Autodesk Fusion 360 part; units mm, degrees
cylinder "CylinderPrimitive1" add diameter 18.6 height 24.7 placed x (1, 0, 0) y (0, 0, -1) z (0, 1, 0) at (0, 0, 0)
hole "Hole1" at (0, 24.7, 0) direction (0, -1, 0) diameter 8 depth 10 tip angle 180
hole "Hole2" at (0, 0, 0) direction (0, 1, 0) diameter 4.7 depth 10 tip angle 180
Build history of the part. All positions in model axes, mm. A direction names the side the tool comes from. Coordinates: 2 decimals unless noted, no trailing zeros. Order: outer loops, then holes, each group sorted by start corner. A loop starts at its lowest first (then second) coordinate and runs counter-clockwise, first axis right, second up. Notation, with made-up numbers: M -2,47 L 33,47 A17 ccw 33,68 Z; hole C 19.25,-1.5 d3. An arc over 180 degrees is marked long. One line per question, with ' | ' between items. Start each with the question number.
Q1. Two-plate mould, pull along X, no slides. Class faces 1 (the face through (2, 0, 2)), 2 (the face through (0, 14.7, 0)), 3 (the face through (5, 12.52, -7.84)): +X half, -X half, draft (parallel to the pull), parting line (faces both ways), or undercut.
Q2. Saw through at B-B (z = 0). List the corners of the cut face in (x, y), then the cut area to 3 significant figures.
Q3. Saw through at C-C (y = 6). List the corners of the cut face in (x, z).
Q4. 3-axis set-ups, long thin cutter, end or side, ignore diameter. For faces 4 (the face through (4, 24.7, 2)), 5 (the face through (3.905, 19.63, -0.867)), 6 (the face through (2.294, 5.07, 0.509)): which of +Z, -Z, +X, -X, +Y, -Y reach the whole face in a straight line?
Q5. Probe L1, parallel to X at y = 18.25, z = 0; L2, parallel to Z at x = 0, y = 4.25. List the from-to ranges inside material, lowest first. Write a range as from..to.
Q6. Saw through at A-A (x = 0). List the corners of the cut face in (y, z), then the cut area to 3 significant figures.
Q7. Saw through at D-D (y = 14). List the corners of the cut face in (x, z).
Q8. Flat gauge pins, fed straight in: pin 1 Ø6 at (x, z) = (0, 0) entering from +Y; pin 2 Ø4 at (y, z) = (12, -5) entering from -X; pin 3 Ø6 at (y, z) = (7.5, 7) entering from +X. Where does each tip first touch, or does it go through?
Check values:
1) face 1: draft | face 2: undercut | face 3: parting line
2) outline: M -9.3,0 L -2.35,0 L -2.35,10 L 2.35,10 L 2.35,0 L 9.3,0 L 9.3,24.7 L 4,24.7 L 4,14.7 L -4,14.7 L -4,24.7 L -9.3,24.7 Z | area: 332 mm2
3) outline: C 0,0 d18.6; hole C 0,0 d4.7
4) face 4: +Z, -Z, +X, -X, +Y | face 5: +Y | face 6: -Y
5) L1: x = -9.3..-4, 4..9.3 | L2: z = -9.3..-2.35, 2.35..9.3
6) outline: M 0,-9.3 L 24.7,-9.3 L 24.7,-4 L 14.7,-4 L 14.7,4 L 24.7,4 L 24.7,9.3 L 0,9.3 L 0,2.35 L 10,2.35 L 10,-2.35 L 0,-2.35 Z | area: 332 mm2
7) outline: C 0,0 d18.6
8) pin 1: stops at y = 14.7 | pin 2: stops at x = -8.8 | pin 3: stops at x = 8.4
